For this review, take the finished solid that the model builds, in its own axes (mm). Face numbers are marked on the shaded views. A direction names the side the tool comes from. Give positions to 0.01 mm unless a question says otherwise; leave off trailing zeros. Write each loop counter-clockwise with the first axis right and the second up, starting at its lowest first coordinate (ties: lowest second). Pieces come first, ordered by that corner, then holes.
Q1. We need section B-B (x = 0.5). Write out the cut boundary in (y, z), then the cut area to 3 significant figures.
Q2. We need section A-A (z = 0). Write out the cut boundary in (x, y), then the cut area to 4 significant figures.
Q3. For line 1 (Y direction, x = 10.8, z = 0); line 2 (X direction, y = 20, z = -3.5); line 3 (Z direction, x = 10.65, y = 8), list the stretches that pass through material, from the lowest coordinate up.
Q4. Machinability: for the marked faces 1, 2, 3 and 4, which of the approach directions +Z, -Z, +X, -X, +Y, -Y give a long, thin tool a straight path to every point of the face, cutting with its end or side? Answer none if there is none.
Q5. Insertion check: P1, Ø3, axis at y = 7.5, z = -1.5, coming from the +X side; P2, Ø2, axis at y = 9, z = -8, coming from the -X side; P3, Ø2, axis at x = -2.5, y = 15.5, coming from the +Z side. Each pin has a flat end and moves straight along its axis. Give the tip position at first contact, or say it passes through.
Q6. Mouldability with a two-part tool opening along X and no side actions: class the marked faces 5, 6 and 7 as released by +X, released by -X, zero draft, split by the parting line, or undercut.
Autodesk Inventor part; units mm, degrees
ref_plane "YZ Plane" through (0, 0, 0) normal (1, 0, 0) x (0, 1, 0)
ref_plane "XZ Plane" through (0, 0, 0) normal (0, 1, 0) x (-1, 0, 0)
ref_plane "XY Plane" through (0, 0, 0) normal (0, 0, 1) x (1, 0, 0)
sketch "Эскиз1" plane through (0, 0, 0) normal (0, 1, 0) x (-1, 0, 0)
  circle A0 centre (0, 0) radius 3.95
  circle A1 centre (0, 0) radius 4.95
  line L0 (0, 0) -> (3.95, 2.9833)
  line L1 (0, 0) -> (3.95, -2.9833)
  point P0 (3.152, -2.3806)
  point P1 (3.152, 2.3806)
  dimension "d0" = 7.9
  dimension "d1" = 9.9
extrude "Выдавливание1" add sketch "Эскиз1" along normal blind 30 contours A0 L1 A1 L0 picked at (3.1693, 3.3115)
sketch "Эскиз2" plane through (0, 30, 0) normal (0, 1, 0) x (1, 0, 0)
  arc A0 (-3.152, -2.3806) -> (-3.152, 2.3806) centre (0, 0) ccw
  arc A1 (-3.152, -2.3806) -> (-4.0447, -1.8507) centre (-5.8533, -5.9145) ccw
  arc A2 (-4.0447, -1.8507) -> (-5.2016, -3.6565) centre (-4.4791, -2.8459) ccw
  line L0 (-5.2016, -3.6565) -> (-4.5303, -2.802)
  arc A3 (-3.9514, -2.9687) -> (-4.5303, -2.802) centre (-4.3197, -3.1592) ccw
  line L1 (0, 0) -> (-3.2711, 0)
  arc A4 (-4.0447, 1.8507) -> (-3.152, 2.3806) centre (-5.8533, 5.9145) ccw
  arc A5 (-5.2016, 3.6565) -> (-4.0447, 1.8507) centre (-4.4791, 2.8459) ccw
  line L2 (-5.2016, 3.6565) -> (-4.5303, 2.802)
  arc A6 (-4.5303, 2.802) -> (-3.9514, 2.9687) centre (-4.3197, 3.1592) ccw
  line L3 (-3.152, -2.3806) -> (-3.95, -2.9833)
  line L4 (-3.95, -2.9833) -> (-3.152, -2.3806)
  line L5 (-3.95, -2.9833) -> (-3.9514, -2.9687)
  line L6 (-3.152, 2.3806) -> (-3.95, 2.9833)
  line L7 (-3.95, 2.9833) -> (-3.9514, 2.9687)
extrude "Выдавливание2" add sketch "Эскиз2" against normal blind 30
sketch "Эскиз3" plane through (0, 30, 0) normal (0, 1, 0) x (1, 0, 0)
  arc A0 (-3.95, -2.9833) -> (-3.95, 2.9833) centre (0, 0) ccw
  line L0 (11.5, -5.45) -> (11.5, 5.45)
  arc A1 (-3.152, -2.3806) -> (-3.152, 2.3806) centre (0, 0) ccw
  arc A2 (0, -3.95) -> (0, 3.95) centre (0, 0) ccw
  line L1 (0, -4.95) -> (0, -3.95)
  line L2 (0, 3.95) -> (0, 4.95)
  line L3 (11.5, 5.45) -> (11.5, 9.45)
  line L4 (11.5, -5.45) -> (11.5, -9.45)
  line L5 (11.5, 9.45) -> (0, 9.45)
  line L6 (0, 9.45) -> (0, 4.95)
  line L7 (11.5, -9.45) -> (0, -9.45)
  line L8 (0, -9.45) -> (0, -4.95)
  dimension "d13" = 4
  dimension "d14" = 4
  dimension "d21" = 11.5
  dimension "d22" = 18.9
  dimension "d23" = 5.5
extrude "Выдавливание3" add sketch "Эскиз3" against normal blind 30 contours A0 L6 L5 L3 L0 L4 L7 L8
sketch "Эскиз4" plane through (11.5, 20, 4.95) normal (1, 0, 0) x (0, 0, -1)
  line L0 (4.95, -20) -> (4.95, 10)
  line L1 (1, 10) -> (8.9, 10)
  circle A0 centre (4.95, -12) radius 5
  line L2 (14.4, -20) -> (-4.5, -20)
  circle A1 centre (4.95, 2) radius 5
  line L3 (-4.5, 10) -> (14.4, 10)
  point P0 (7.3306, 10)
  point P1 (2.5694, 10)
  point P2 (4.95, 10)
  dimension "d15" = 10
  dimension "d16" = 8
  dimension "d17" = 10
  dimension "d18" = 8
extrude "Выдавливание4" cut sketch "Эскиз4" against normal blind 2
properties part number "крепление маркера"
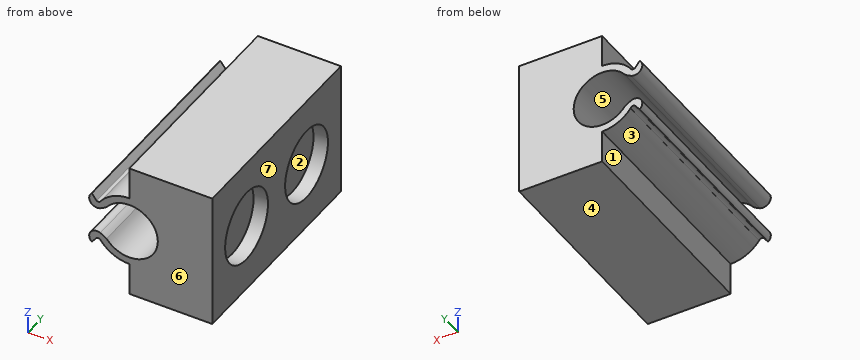
Computed:
1. outline: (0, -9.45) - (30, -9.45) - (30, -3.92) - (0, -3.92) - close; (0, 3.92) - (30, 3.92) - (30, 9.45) - (0, 9.45) - close
1. area: 332 mm2
2. outline: (3.95, 0) - (11.5, 0) - (11.5, 3) - (9.5, 3) - (9.5, 13) - (11.5, 13) - (11.5, 17) - (9.5, 17) - (9.5, 27) - (11.5, 27) - (11.5, 30) - (3.95, 30) - close
2. area: 186.5 mm2
3. line 1: y = 0 to 3, 13 to 17, 27 to 30
3. line 2: x = -5.35 to -5.08, -3.5 to -1.83, 1.83 to 9.5
3. line 3: z = -9.45 to -5, 5 to 9.45
4. face 1: -Z, -X, +Y, -Y
4. face 2: +X
4. face 3: -Z, +Y, -Y
4. face 4: -Z, +X, -X, +Y, -Y
5. P1: stops at x = 9.5
5. P2: stops at x = 0
5. P3: stops at z = 4.72
6. face 5: undercut
6. face 6: zero draft
6. face 7: released by +X
